Autodesk Inventor part; units mm, degrees
ref_plane "YZ Plane" through (0, 0, 0) normal (1, 0, 0) x (0, 1, 0)
ref_plane "XZ Plane" through (0, 0, 0) normal (0, 1, 0) x (-1, 0, 0)
ref_plane "XY Plane" through (0, 0, 0) normal (0, 0, 1) x (1, 0, 0)
sketch "Sketch1" plane through (0, 0, 0) normal (0, 0, 1) x (1, 0, 0)
  line L0 (0, 0) -> (0, 6)
  line L1 (0, 6) -> (5, 6)
  line L2 (5, 6) -> (5, 0)
  line L3 (5, 0) -> (3.5, 0)
  line L4 (3.5, 0) -> (3.5, 3)
  line L5 (3.5, 3) -> (0, 3)
  point P0 (4.25, 0)
  dimension "d0" = 7
  dimension "d1" = 10
  dimension "d2" = 3
  dimension "d3" = 6
revolve "Revolution1" add sketch "Sketch1" angle 360 about axis through (0, 0, 0) along (0, 1, 0)
sketch "Sketch2" plane through (0, 3, 0) normal (0, -1, 0) x (1, 0, 0)
  circle A0 centre (0, 0) radius 3.5
hole "Hole1" at (0, 3, 0) direction (0, 1, 0) diameter 3 depth 3 countersink diameter 6 countersink angle 90
fillet "Fillet1" radius 1 1 edges at (-5, 6, 0)
properties part number "26b"
Geometry: final body of the model. Coordinates: model frame, mm. A direction names the side the tool comes from. Round coordinates to 2 decimals unless told otherwise and drop trailing zeros. Order: outer loops, then holes, each group sorted by start corner. A loop starts at its lowest first (then second) coordinate and runs counter-clockwise, first axis right, second up.
Q1. Section A-A, the plane x = 0. Output: boundary loops of the cut face in (y, z).
Result sheet:
outline: (0, -5) - (5, -5) arc R1 ccw to (6, -4) - (6, -1.5) - (4.5, -1.5) - (3, -3) - (3, -3.5) - (0, -3.5) - close; (0, 3.5) - (3, 3.5) - (3, 3) - (4.5, 1.5) - (6, 1.5) - (6, 4) arc R1 ccw to (5, 5) - (0, 5) - close
Q2. Section B-B, the plane z = 0. Output: boundary loops of the cut face in (x, y).
Result sheet:
outline: (-5, 0) - (-3.5, 0) - (-3.5, 3) - (-3, 3) - (-1.5, 4.5) - (-1.5, 6) - (-4, 6) arc R1 ccw to (-5, 5) - close; (1.5, 4.5) - (3, 3) - (3.5, 3) - (3.5, 0) - (5, 0) - (5, 5) arc R1 ccw to (4, 6) - (1.5, 6) - close
Q3. Material intervals for probe 1 along Z at (x, y) = (0, 1.8); probe 2 along Z at (x, y) = (0, 4.95), sorted ascending.
Result sheet:
probe 1: z = -5 to -3.5, 3.5 to 5
probe 2: z = -5 to -1.5, 1.5 to 5
Q4. Mould query, pull axis X, two halves, no side actions, for faces 1 (the face through (3, 3, -1)), 2 (the face through (2.2, 0, 3.3)), 3 (the face through (-1.08, 2.46, -4.88)). Classes: released by +X, released by -X, zero draft, split by the parting line, or undercut.
Result sheet:
face 1: undercut
face 2: zero draft
face 3: split by the parting line
Q5. Section C-C, the plane y = 0.5. Output: boundary loops of the cut face in (x, z).
Result sheet:
outline: circle Ø10 at (0, 0); hole circle Ø7 at (0, 0)
Q6. Access query for faces 4 (the face through (3.233, 1.521, 1.341)), 5 (the face through (2, 6, 0)). Directions: +Z, -Z, +X, -X, +Y, -Y. A direction counts if a zero-diameter tool reaches every point of the face in a straight line with its end or side. Return the directions, or none.
Result sheet:
face 4: -Y
face 5: +Z, -Z, +X, -X, +Y
